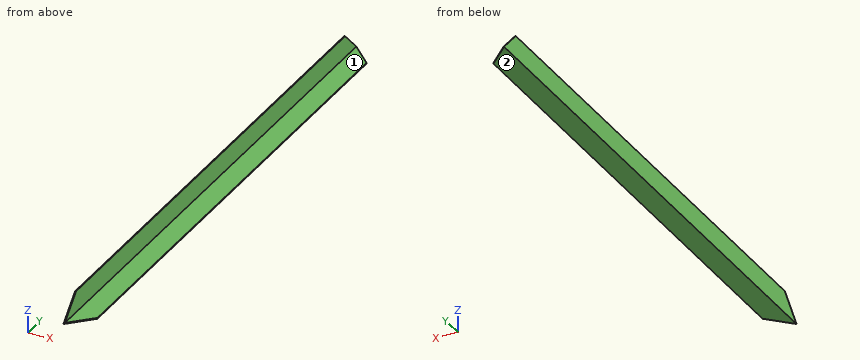
from build123d import *

# Parameters (mm, degrees)
AUFSATZ_LINEAR_AUSTRAGEN1_DEPTH      = 499.9
AUFSATZ_LINEAR_AUSTRAGEN1_DEPTH_BACK = 499.9
SCHNITT_LINEAR_AUSTRAGEN1_DEPTH      = 1.5
SCHNITT_LINEAR_AUSTRAGEN2_DEPTH      = 1.5


with BuildPart() as part:
    # Skizze1 → Aufsatz-Linear austragen1 (new, two sides: drawn at the far end of the back side and taken through both)
    with BuildSketch(Plane(origin=(0, 0, 0), x_dir=(1, 0, 0), z_dir=(0, 1, 0)).offset(-AUFSATZ_LINEAR_AUSTRAGEN1_DEPTH_BACK)):
        Polygon((-461.5, 4), (-461.5, 5.5), (-501.5, 5.5), (-501.5, -34.5), (-500, -34.5), (-500, 4), align=None)
    extrude(amount=AUFSATZ_LINEAR_AUSTRAGEN1_DEPTH + AUFSATZ_LINEAR_AUSTRAGEN1_DEPTH_BACK)

    # Skizze2 → Schnitt-Linear austragen1 (cut)
    with BuildSketch(Plane(origin=(0, 0, -5.5), x_dir=(-1, 0, 0), z_dir=(0, 0, -1))):
        Polygon((501.5, 499.9), (461.5, 459.9), (461.5, 499.9), align=None)
        Polygon((461.5, -459.9), (461.5, -499.9), (501.5, -499.9), align=None)
    extrude(amount=-SCHNITT_LINEAR_AUSTRAGEN1_DEPTH, mode=Mode.SUBTRACT)

    # Skizze3 → Schnitt-Linear austragen2 (cut)
    with BuildSketch(Plane.ZY.offset(501.5)):
        Polygon((34.5, 499.9), (-5.5, 499.9), (34.5, 459.9), align=None)
        Polygon((-5.5, -499.9), (34.5, -459.9), (34.5, -499.9), align=None)
    extrude(amount=-SCHNITT_LINEAR_AUSTRAGEN2_DEPTH, mode=Mode.SUBTRACT)


solid = part.part
The listing builds one solid part. Answer for the finished solid, in the listing's coordinates (mm). Face numbers are marked on the shaded views. A direction names the side the tool comes from. Round coordinates to 2 decimals unless told otherwise and drop trailing zeros. Order: outer loops, then holes, each group sorted by start corner. A loop starts at its lowest first (then second) coordinate and runs counter-clockwise, first axis right, second up. Notation, with made-up numbers: (29.5, -1.75) -> (74.5, -1.75) arc R9 cw to (74.5, 11.25) -> close; hole circle Ø1 at (17, -37). An arc over 180 degrees is marked (long way). Put each result on its own line as item: value.
Q1. Which of the six approach directions +Z, -Z, +X, -X, +Y, -Y give full straight-line access (tool end or side, diameter ignored) to the marked faces 1 and 2?
Results list:
face 1: +Z, +X, +Y, -Y
face 2: -Z, +X, -X, +Y, -Y
Q2. Section A-A, the plane x = -490 is taken. Write down the section's boundary in (y, z).
Results list:
outline: (-488.4, -5.5) -> (488.4, -5.5) -> (488.4, -4) -> (-488.4, -4) -> close
Q3. This flat-tipped pin is pushed along its axis until it touches: P1, Ø10, axis at x = -471, y = 258.5, coming from the +Z side. Where does it stop, or does it pass through?
Results list:
P1: z = -4
Q4. Section C-C, the plane y = 420 is taken. Write down the section's boundary in (x, z).
Results list:
outline: (-501.5, -5.5) -> (-461.5, -5.5) -> (-461.5, -4) -> (-500, -4) -> (-500, 34.5) -> (-501.5, 34.5) -> close
Q5. Consider line 1 along Z through (x, y) = (-495, -346.5); line 2 along X through (y, z) = (-121, -3.5). Determine where each line is inside the solid, lowest interval first.
Results list:
line 1: -5.5 to -4
line 2: -501.5 to -500
Q6. Section B-B, the plane z = 21.5 is taken. Write down the section's boundary in (x, y), and give its area (3 significant figures).
Results list:
outline: (-501.5, -472.9) -> (-500, -472.9) -> (-500, 472.9) -> (-501.5, 472.9) -> close
area: 1,420 mm^2
